Geometry: final body of the model. Coordinates: model frame, mm. Face numbers are marked on the shaded views. A direction names the side the tool comes from. Give positions to 0.01 mm unless a question says otherwise; leave off trailing zeros. Write each loop counter-clockwise with the first axis right and the second up, starting at its lowest first coordinate (ties: lowest second). Pieces come first, ordered by that corner, then holes. Notation, with made-up numbers: (23.5, -5.75) - (47.5, -5.75) arc R22 ccw to (47.5, 10.25) - close; hole circle Ø8 at (-35.75, 68). An arc over 180 degrees is marked (long way). Use CSV: the item, a comma, the result in double quotes. Start each with the question number.
(1) Section B-B on x = 20.5. Output: boundary loops of the cut face in (y, z).
(2) Line query: probe 1 along Z at (x, y) = (19.5, 3). Output: solid intervals per line, ascending. Write a range as [from, to].
(3) First-contact query: pin 1 Ø5 at (x, y) = (17.5, 4.5) entering from +Z; pin 2 Ø5 at (x, y) = (22.5, 5.5) entering from -Z. Flat tips, straight axial feed; report the tip coordinate or a pass-through.
(4) Reachability of the marked faces 1, 2 and 3 from +Z, -Z, +X, -X, +Y, -Y: full face, straight path, thin tool, end or side. Return the list, or none.
(5) Section A-A on y = 5.25. Output: boundary loops of the cut face in (x, z), and give its area (3 significant figures).
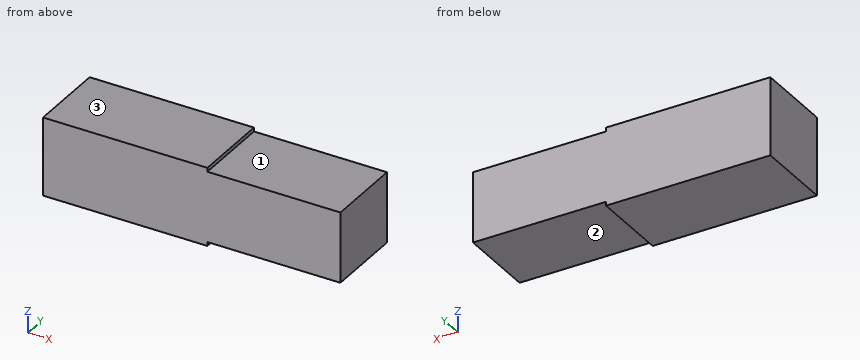
from build123d import *

# Parameters (mm, degrees)
SKETCH_1_W      = 21
SKETCH_1_H      = 10
SKETCH_1_W_2    = 17
SKETCH_1_H_2    = 9
EXTRUDE_1_DEPTH = 10


with BuildPart() as part:
    # 草图1 → 凸台-拉伸1 (new body)
    with BuildSketch(Plane(origin=(0, 0, 0), x_dir=(1, 0, 0), z_dir=(0, 1, 0))):
        Rectangle(SKETCH_1_W, SKETCH_1_H)
        with Locations((19, 0)):
            Rectangle(SKETCH_1_W_2, SKETCH_1_H_2)
    extrude(amount=EXTRUDE_1_DEPTH)


solid = part.part
Check values:
1,outline,"(0, -4.5) - (10, -4.5) - (10, 4.5) - (0, 4.5) - close"
2,probe 1,"z = [-4.5, 4.5]"
3,pin 1,"stops at z = 4.5"
3,pin 2,"stops at z = -4.5"
4,face 1,"+Z, +X, +Y, -Y"
4,face 2,"-Z, +X, +Y, -Y"
4,face 3,"+Z, +X, -X, +Y, -Y"
5,outline,"(-10.5, -5) - (10.5, -5) - (10.5, -4.5) - (27.5, -4.5) - (27.5, 4.5) - (10.5, 4.5) - (10.5, 5) - (-10.5, 5) - close"
5,area,"363 mm²"
